```python
from build123d import *

# Parameters (mm, degrees)
SKETCH_1_R          = 1.6
EXTRUDE_1_DEPTH     = 5
EXTRUDE_START       = -10
EXTRUDE_2_DEPTH     = 18
SKETCH_4_W          = 10
SKETCH_4_H          = 18
EXTRUDE_3_DEPTH     = 6.14228691
SKETCH_5_R          = 2
CUT_EXTRUDE_1_DEPTH = 5


with BuildPart() as part:
    # 草图1 → 凸台-拉伸1 (new body)
    with BuildSketch(Plane.XY):
        Polygon((0, 0), (0, 38), (10, 38), (10, 22.5), (28, 22.5), (28, 38), (38, 38), (38, 0), (28, 0), (28, 15.5), (10, 15.5), (10, 0), align=None)
        with Locations((5, 33)):
            Circle(SKETCH_1_R, mode=Mode.SUBTRACT)
        with Locations((33, 33)):
            Circle(SKETCH_1_R, mode=Mode.SUBTRACT)
        with Locations((33, 5)):
            Circle(SKETCH_1_R, mode=Mode.SUBTRACT)
        with Locations((5, 5)):
            Circle(SKETCH_1_R, mode=Mode.SUBTRACT)
    extrude(amount=EXTRUDE_1_DEPTH)

    # 草图2 → 凸台-拉伸2 (add)
    with BuildSketch(Plane(origin=(38, 0, 0), x_dir=(0, 0, -1), z_dir=(1, 0, 0)).offset(EXTRUDE_START)):
        Polygon((0, 22.5), (20, 27.133580113), (30.962428796, 37.371995756), (35.154914556, 32.883036896), (22, 20.596938124), (0, 15.5), align=None)
    extrude(amount=-EXTRUDE_2_DEPTH)

    # 草图4 → 凸台-拉伸3 (add)
    with BuildSketch(Plane(origin=(0, 0.026666642, 0.024905444), x_dir=(1, 0, 0), z_dir=(0, -0.7308285864179805, -0.682561042892353))):
        with Locations((5, -39.136896468)):
            Rectangle(SKETCH_4_W, SKETCH_4_H)
        with Locations((33, -39.136896468)):
            Rectangle(SKETCH_4_W, SKETCH_4_H)
    extrude(amount=-EXTRUDE_3_DEPTH)

    # 草图5 → 切除-拉伸1 (cut)
    with BuildSketch(Plane(origin=(0, 0.026666642, 0.024905444), x_dir=(1, 0, 0), z_dir=(0, -0.7308285864179805, -0.682561042892353))):
        with Locations(Location((5, -43.136896468, 0), (0, 0, 270))):
            Circle(SKETCH_5_R)
        with Locations(Location((33, -43.136896468, 0), (0, 0, 270))):
            Circle(SKETCH_5_R)
    extrude(amount=-CUT_EXTRUDE_1_DEPTH, mode=Mode.SUBTRACT)


solid = part.part
```
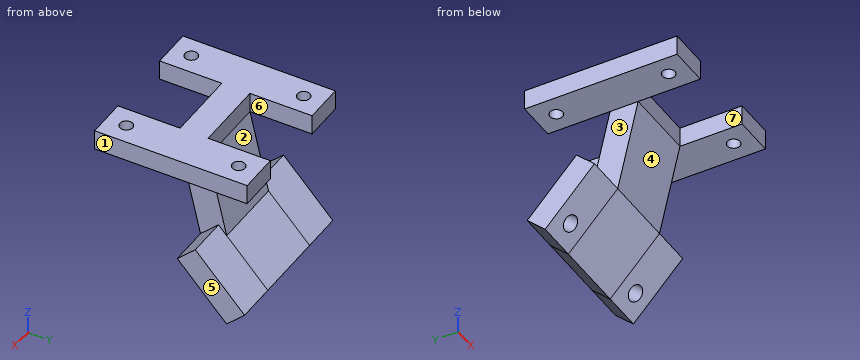
Check sheet for the modelled part. Datum: model origin and axes. Units: mm. Face numbers are marked on the shaded views. A direction names the side the tool comes from. Give positions to 0.01 mm unless a question says otherwise; leave off trailing zeros. Order: outer loops, then holes, each group sorted by start corner. A loop starts at its lowest first (then second) coordinate and runs counter-clockwise, first axis right, second up. Notation, with made-up numbers: M 13.25,19.5 L 43.25,19.5 A19 cw 43.25,46.5 Z; hole C -34.75,89.5 d2. An arc over 180 degrees is marked long. Answer in a Markdown table with one row per item. Add a question column.
Q1. Thickness scan on L1, parallel to Y at x = 33, z = 1.55; L2, parallel to X at y = 33, z = -29; L3, parallel to Z at x = 5.5, y = 3. Record the ranges inside material, lowest first.
Q2. Access from +Z, -Z, +X, -X, +Y, -Y to the whole of each face (thin tool, end or side, straight path). Record for the marked faces 5, 6 and 7.
Q3. Release check for a two-part mould opening along Z. For the marked faces 1, 2, 3 and 4 record: released by +Z, released by -Z, zero draft, split by the parting line, or undercut.
Q4. Gauge pin test, flat ends, axial feed: pin 1 Ø4 at (x, z) = (22.5, 1.5) entering from +Y; pin 2 Ø9.5 at (y, z) = (19.5, -7.5) entering from +X; pin 3 Ø3 at (x, y) = (8, 16.5) entering from -Z; pin 4 Ø2.5 at (x, y) = (33, 33) entering from -Z. Record the tip position at first contact, or that the pin passes through.
Q5. Sectioned sample at B-B, the plane x = 29.5. Record the boundary of the cut face in (y, z), and give its area (3 significant figures).
Q6. Sectioned sample at A-A, the plane y = 5. Record the boundary of the cut face in (x, z), and give its area (3 significant figures).
Q7. Sectioned sample at C-C, the plane x = 5. Record the boundary of the cut face in (y, z).
Q8. Sectioned sample at D-D, the plane x = 11.5. Record the boundary of the cut face in (y, z), and give its area (3 significant figures).
Verdict:
| question | item | result |
|---|---|---|
| 1 | L1 | 0 to 3.4, 6.6 to 31.4, 34.6 to 38 |
| 1 | L2 | 0 to 3.09, 6.91 to 31.09, 34.91 to 38 |
| 1 | L3 | 0 to 5 |
| 2 | face 5 | +Z, -Z, +X, +Y, -Y |
| 2 | face 6 | +Z, +Y |
| 2 | face 7 | +Z, -Z, -Y |
| 3 | face 1 | zero draft |
| 3 | face 2 | released by +Z |
| 3 | face 3 | undercut |
| 3 | face 4 | released by -Z |
| 4 | pin 1 | y = 22.62 |
| 4 | pin 2 | x = 28 |
| 4 | pin 3 | z = 0 |
| 4 | pin 4 | z = -35.15 |
| 5 | outline | M 0,0 L 38,0 L 38,5 L 0,5 Z; M 20.6,-22 L 32.88,-35.15 L 37.37,-30.96 L 25.09,-17.81 Z |
| 5 | area | 301 mm² |
| 6 | outline | M 0,0 L 3.4,0 L 3.4,5 L 0,5 Z; M 6.6,0 L 10,0 L 10,5 L 6.6,5 Z; M 28,0 L 31.4,0 L 31.4,5 L 28,5 Z; M 34.6,0 L 38,0 L 38,5 L 34.6,5 Z |
| 6 | area | 68.0 mm² |
| 7 | outline | M 0,0 L 3.4,0 L 3.4,5 L 0,5 Z; M 6.6,0 L 31.4,0 L 31.4,5 L 6.6,5 Z; M 20.6,-22 L 28.11,-30.04 L 31.76,-26.63 L 34.49,-29.55 L 30.84,-32.96 L 32.88,-35.15 L 37.37,-30.96 L 25.09,-17.81 Z; M 34.6,0 L 38,0 L 38,5 L 34.6,5 Z |
| 8 | outline | M 15.5,0 L 20.6,-22 L 32.88,-35.15 L 37.37,-30.96 L 27.13,-20 L 22.5,0 L 22.5,5 L 15.5,5 Z |
| 8 | area | 283 mm² |
